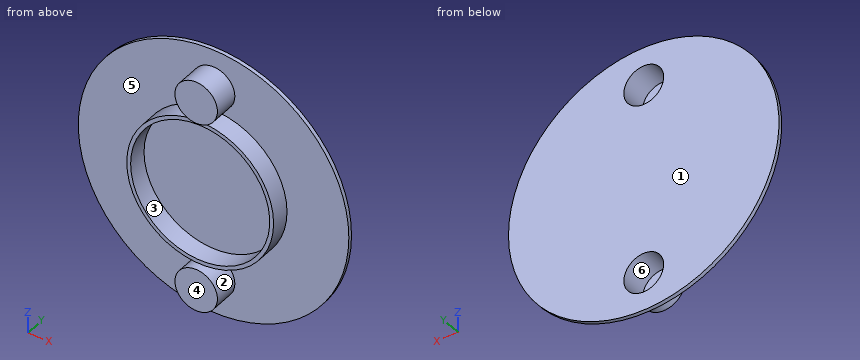
Autodesk Inventor part; units mm, degrees
ref_plane "YZ Plane" through (0, 0, 0) normal (1, 0, 0) x (0, 1, 0)
ref_plane "XZ Plane" through (0, 0, 0) normal (0, 1, 0) x (-1, 0, 0)
ref_plane "XY Plane" through (0, 0, 0) normal (0, 0, 1) x (1, 0, 0)
sketch "Sketch1" plane through (0, 0, 0) normal (0, 1, 0) x (-1, 0, 0)
  circle A0 centre (0, 0) radius 18
  circle A1 centre (0, 0) radius 19
  dimension "d0" = 36
  dimension "d1" = 38
extrude "Extrusion1" add sketch "Sketch1" along normal blind 5
sketch "Sketch2" plane through (0, 5, 0) normal (0, 1, 0) x (1, 0, 0)
  circle A0 centre (0, 0) radius 35
  circle A1 centre (0, 0) radius 19
  circle A2 centre (0, -25) radius 5.15
  circle A3 centre (0, 25) radius 5.15
  dimension "d4" = 16
  dimension "d5" = 10.3
  dimension "d6" = 10.3
  dimension "d7" = 25
  dimension "d8" = 25
extrude "Extrusion2" add sketch "Sketch2" along normal blind 1 contours A0 | A1
sketch "Sketch3" plane through (0, 5, 0) normal (0, -1, 0) x (1, 0, 0)
  circle A0 centre (0, 25) radius 5.15
  circle A1 centre (0, -25) radius 5.15
  circle A2 centre (0, -25) radius 5.15
  circle A3 centre (0, 25) radius 5.15
  circle A4 centre (0, 25) radius 5.5
  circle A5 centre (0, -25) radius 5.5
  point P0 (0, 0)
  point P1 (-4.4822, -18.4638)
  point P2 (4.4822, -18.4638)
  point P3 (4.4822, 18.4638)
  point P4 (-4.4822, 18.4638)
  dimension "d11" = 10.3
  dimension "d12" = 10.3
  dimension "d13" = 0
  dimension "d14" = 0
  dimension "d15" = 11
  dimension "d16" = 11
extrude "Extrusion3" add sketch "Sketch3" along normal blind 6
sketch "Sketch4" plane through (0, -1, 25) normal (0, -1, 0) x (1, 0, 0)
  circle A0 centre (0, 0) radius 5.5
  circle A1 centre (0, -50) radius 5.5
  circle A2 centre (0, -50) radius 5.5
  point P0 (0, -25)
  dimension "d19" = 11
  dimension "d20" = 0
extrude "Extrusion4" add sketch "Sketch4" along normal blind 0.5
properties part number "magnet_holder"
Build history of the part. All positions in model axes, mm. Face numbers are marked on the shaded views. A direction names the side the tool comes from. Coordinates: 2 decimals unless noted, no trailing zeros. Write each loop counter-clockwise with the first axis right and the second up, starting at its lowest first coordinate (ties: lowest second). Pieces come first, ordered by that corner, then holes.
(1) 3-axis set-ups, long thin cutter, end or side, ignore diameter. For the marked faces 4, 5 and 6: which of +Z, -Z, +X, -X, +Y, -Y reach the whole face in a straight line?
(2) Mould opens along X. For the marked faces 1, 2 and 3 say: pulls with the +X half, pulls with the -X half, needs draft (parallel to the pull), parting line crosses it, or undercut.
(3) Drill centre lines: line 1 (Z direction, x = 0, y = 1.25); line 2 (Y direction, x = 8, z = 12); line 3 (Z direction, x = -6.5, y = 1.25). Where is each one in solid material? Low to high.
(4) Pin check, flat tips, straight feed: pin 1 Ø6 at (x, z) = (0, -25) entering from +Y; pin 2 Ø11.5 at (x, z) = (-9.5, -1) entering from -Y; pin 3 Ø1 at (y, z) = (0, -1) entering from +X. Stop position of each tip, or through.
(5) Cut at C-C on x = 12.5. List the corners of the cut face in (y, z).
(6) Cut at D-D on x = 26.5. List the corners of the cut face in (y, z), and give its area (3 significant figures).
(7) Cut at B-B on z = 0. List the corners of the cut face in (x, y), and give its area (3 significant figures).
(8) Cut at A-A on x = 0. List the corners of the cut face in (y, z), and give its area (3 significant figures).
Working result:
1. face 4: +Z, -Z, +X, -X, -Y
1. face 5: -Y
1. face 6: +Y
2. face 1: needs draft
2. face 2: parting line crosses it
2. face 3: undercut
3. line 1: z = -30.5 to -30.15, -19.85 to -19.5, -19 to -18, 18 to 19, 19.5 to 19.85, 30.15 to 30.5
3. line 2: y = 5 to 6
3. line 3: z = -17.85 to -16.79, 16.79 to 17.85
4. pin 1: stops at y = -1
4. pin 2: stops at y = 5
4. pin 3: stops at x = 18.99
5. outline: (0, -14.31) - (5, -14.31) - (5, -32.69) - (6, -32.69) - (6, 32.69) - (5, 32.69) - (5, 14.31) - (0, 14.31) - (0, 12.95) - (5, 12.95) - (5, -12.95) - (0, -12.95) - close
6. outline: (5, -22.86) - (6, -22.86) - (6, 22.86) - (5, 22.86) - close
6. area: 45.7 mm2
7. outline: (-35, 5) - (-19, 5) - (-19, 0) - (-18, 0) - (-18, 5) - (18, 5) - (18, 0) - (19, 0) - (19, 5) - (35, 5) - (35, 6) - (-35, 6) - close
7. area: 80.0 mm2
8. outline: (-1.5, -30.5) - (5, -30.5) - (5, -35) - (6, -35) - (6, -30.15) - (-1, -30.15) - (-1, -19.85) - (6, -19.85) - (6, 19.85) - (-1, 19.85) - (-1, 30.15) - (6, 30.15) - (6, 35) - (5, 35) - (5, 30.5) - (-1.5, 30.5) - (-1.5, 19.5) - (5, 19.5) - (5, 19) - (0, 19) - (0, 18) - (5, 18) - (5, -18) - (0, -18) - (0, -19) - (5, -19) - (5, -19.5) - (-1.5, -19.5) - close
8. area: 78.8 mm2
